Autodesk Inventor part; units mm, degrees
ref_plane "YZ Plane" through (0, 0, 0) normal (1, 0, 0) x (0, 1, 0)
ref_plane "XZ Plane" through (0, 0, 0) normal (0, 1, 0) x (-1, 0, 0)
ref_plane "XY Plane" through (0, 0, 0) normal (0, 0, 1) x (1, 0, 0)
sketch "Sketch1" plane through (0, 0, 0) normal (0, 1, 0) x (-1, 0, 0)
  line L0 (-38.1, 25.4) -> (38.1, 25.4)
  line L1 (38.1, 25.4) -> (38.1, -25.4)
  line L2 (38.1, -25.4) -> (-38.1, -25.4)
  line L3 (-38.1, -25.4) -> (-38.1, 25.4)
  point P0 (0, 0)
  dimension "d0" = 50.8
  dimension "d1" = 76.2
  dimension "d2" = 25.4
  dimension "d3" = 38.1
extrude "Extrusion1" add sketch "Sketch1" along normal blind 25.4
sketch "Sketch2" plane through (38.1, 0, 25.4) normal (1, 0, 0) x (0, 0, -1)
  circle A0 centre (25.4, 38.1) radius 26.9875
  line L0 (0, 0) -> (50.8, 0)
  line L1 (50.8, 0) -> (50.8, 25.4)
  line L2 (0, 25.4) -> (50.8, 25.4)
  line L3 (0, 0) -> (0, 25.4)
  point P0 (25.4, 0)
  dimension "d6" = 53.975
extrude "Extrusion2" cut sketch "Sketch2" against normal through all contours A0 L2 | L2 A0
sketch "Sketch3" plane through (0, 0, 0) normal (0, -1, 0) x (1, 0, 0)
  line L0 (38.1, -25.4) -> (-38.1, -25.4)
  line L1 (19.05, -25.4) -> (-19.05, -25.4)
  line L2 (-19.05, -25.4) -> (-19.05, -38.1)
  line L3 (19.05, -38.1) -> (19.05, -25.4)
  line L4 (12.7, -25.4) -> (-12.7, -25.4)
  line L5 (-12.7, -25.4) -> (-12.7, -31.75)
  line L6 (-12.7, -31.75) -> (12.7, -31.75)
  line L7 (12.7, -31.75) -> (12.7, -25.4)
  line L8 (38.1, -25.4) -> (-38.1, -25.4)
  line L9 (38.1, 25.4) -> (38.1, -25.4)
  line L10 (-38.1, 25.4) -> (38.1, 25.4)
  line L11 (-38.1, -25.4) -> (-38.1, 25.4)
  line L12 (-19.05, -38.1) -> (19.05, -38.1)
  point P0 (0, 0)
  point P1 (12.7, -28.575)
  dimension "d10" = 25.4
  dimension "d11" = 6.35
  dimension "d12" = 6.35
  dimension "d13" = 6.35
  dimension "d14" = 6.35
  dimension "d16" = 12.7
extrude "Extrusion3" add sketch "Sketch3" against normal blind 25.4 contours L3 L12 L2 L0 L5 L6 L7
sketch "Sketch4" plane through (19.05, 0, -25.4) normal (1, 0, 0) x (0, 0, -1)
  line L0 (12.7, 0) -> (0, 0)
  line L1 (12.7, 0) -> (12.7, 25.4)
  line L2 (0, 25.4) -> (12.7, 25.4)
  line L3 (0, 0) -> (0, 25.4)
  arc A0 (-49.2125, 25.4) -> (-1.5875, 25.4) centre (-25.4, 38.1) ccw
  line L4 (-50.8, 25.4) -> (-49.2125, 25.4)
  line L5 (-50.8, 0) -> (-50.8, 25.4)
  line L6 (-50.8, 0) -> (0, 0)
  line L7 (0, 0) -> (0, 25.4)
  line L8 (-1.5875, 25.4) -> (0, 25.4)
  line L9 (6.35, 0) -> (0, 0)
  line L10 (0, 0) -> (12.7, 19.05)
  line L11 (12.7, 0) -> (12.7, 25.4)
  point P0 (-25.4, 0)
  point P1 (12.7, 19.05)
  dimension "d19" = 6.35
extrude "Extrusion4" cut sketch "Sketch4" against normal through all contours L0 L10 L1
mirror "Mirror1" about plane through (0, 0, 0) normal (0, 0, 1) of "Extrusion3", "Extrusion4"
sketch "Sketch5" plane through (0, 0, 0) normal (0, -1, 0) x (1, 0, 0)
  line L0 (-12.7, 25.4) -> (-19.05, 25.4)
  line L1 (-38.1, 25.4) -> (-19.05, 25.4)
  line L2 (-38.1, -25.4) -> (-38.1, 25.4)
  line L3 (-19.05, -25.4) -> (-38.1, -25.4)
  line L4 (-19.05, -25.4) -> (-12.7, -25.4)
  line L5 (12.7, -25.4) -> (-12.7, -25.4)
  line L6 (12.7, -25.4) -> (19.05, -25.4)
  line L7 (38.1, -25.4) -> (19.05, -25.4)
  line L8 (38.1, 25.4) -> (38.1, -25.4)
  line L9 (19.05, 25.4) -> (38.1, 25.4)
  line L10 (19.05, 25.4) -> (12.7, 25.4)
  line L11 (-12.7, 25.4) -> (12.7, 25.4)
  line L12 (38.1, 25.4) -> (38.1, 23.8125)
  line L13 (38.1, 25.4) -> (38.1, 31.75)
  line L14 (19.05, 25.4) -> (38.1, 25.4)
  line L15 (29.0711, 25.4) -> (29.0711, 31.75)
  line L16 (-38.1, -25.4) -> (-38.1, -23.8125)
  line L17 (-38.1, -25.4) -> (-38.1, -31.75)
  line L18 (-23.7998, -25.4) -> (-23.7998, -31.75)
  circle A0 centre (-30.9499, -31.75) radius 3.302
  arc A1 (-38.1, -31.75) -> (-23.7998, -31.75) centre (-30.9499, -31.75) ccw
  point P0 (0, 0)
  dimension "d23" = 14.3002
  dimension "d24" = 6.35
  dimension "d25" = 6.35
  dimension "d26" = 6.604
  dimension "d27" = 6.35
  dimension "d28" = 7.1501
  dimension "d29" = 6.35
extrude "Extrusion5" add sketch "Sketch5" against normal blind 6.35 contours L3 L18 A1 L17
mirror "Mirror2" about plane through (0, 0, 0) normal (0, 0, 1) of "Extrusion5"
equation "\"d12\" = d11"
equation "\"d13\" = d11"
equation "\"d25\" = d24"
equation "\"d27\" = d24"
equation "\"d28\" = 0.5 * d23"
equation "\"d29\" = d24"
properties part number "Part_4_scooter_attachment"
Build history of the part. All positions in model axes, mm. A direction names the side the tool comes from. Round coordinates to 2 decimals unless told otherwise and drop trailing zeros. Write each loop counter-clockwise with the first axis right and the second up, starting at its lowest first coordinate (ties: lowest second). Pieces come first, ordered by that corner, then holes.
1) 3-axis set-ups, long thin cutter, end or side, ignore diameter. For faces 4 (the flat face through (0.267, 11.775, 33.25)), 5 (the flat face through (-12.7, 15, 29)), 6 (the flat face through (-23.8, 3, 29)), 7 (the flat face through (19.05, 15, -30)): which of +Z, -Z, +X, -X, +Y, -Y reach the whole face in a straight line?
2) Drill centre lines: probe 1 along X at (y, z) = (4.25, 31.75); probe 2 along X at (y, z) = (3, -26); probe 3 along X at (y, z) = (9.25, -29). Where is each one in solid material? Low to high.
3) Band-saw the part on D-D, the plane z = 30.5. List the corners of the cut face in (x, y), and give its area (3 significant figures).
4) Band-saw the part on B-B, the plane x = -8. Give the number of separate pieces and of enclosed holes in the cut face, and give its area (3 significant figures).
5) Pin check, flat tips, straight feed: pin 1 (3 mm diameter, centred on y = 16.5, z = -27, fed in from +X); pin 2 (6 mm diameter, centred on x = 8.5, y = 10, fed in from +Z); pin 3 (8 mm diameter, centred on x = 1.5, y = 14, fed in from +Z); pin 4 (5 mm diameter, centred on y = 10.5, z = 27.5, fed in from +X). Stop position of each tip, or through.
6) Mould opens along X. For faces 1 (the flat face through (38.1, 10, 0)), 2 (the flat face through (28, 13, -25.4)), 3 (the flat face through (-12.7, 15, -29)) say: +X half, -X half, draft (parallel to the pull), parting line (faces both ways), or undercut.
7) Band-saw the part on A-A, the plane y = 17.75. List the corners of the cut face in (x, z).
Ans:
1. face 4: +Z, +X, -Y
1. face 5: +Y, -Y
1. face 6: +Z, +Y, -Y
1. face 7: -Z, +X, +Y, -Y
2. probe 1: x = -38.1 to -34.25, -27.65 to -23.8
2. probe 2: x = -38.1 to -23.8, -19.05 to -12.7, 12.7 to 19.05
2. probe 3: x = -19.05 to -12.7, 12.7 to 19.05
3. outline: (-38.1, 0) - (-34.01, 0) - (-34.01, 6.35) - (-38.1, 6.35) - close; (-27.89, 0) - (-23.8, 0) - (-23.8, 6.35) - (-27.89, 6.35) - close; (-19.05, 7.65) - (-12.7, 7.65) - (-12.7, 25.4) - (-19.05, 25.4) - close; (12.7, 7.65) - (19.05, 7.65) - (19.05, 25.4) - (12.7, 25.4) - close
3. area: 277 mm2
4. separate pieces: 3
4. enclosed holes: 0
4. area: 947 mm2
5. pin 1: stops at x = 19.05
5. pin 2: stops at z = 34.07
5. pin 3: stops at z = 37.4
5. pin 4: stops at x = 38.1
6. face 1: +X half
6. face 2: draft
6. face 3: undercut
7. outline: (-38.1, -25.4) - (-19.05, -25.4) - (-19.05, -37.23) - (19.05, -37.23) - (19.05, -25.4) - (38.1, -25.4) - (38.1, -17.73) - (-38.1, -17.73) - close; (-38.1, 17.73) - (38.1, 17.73) - (38.1, 25.4) - (19.05, 25.4) - (19.05, 37.23) - (-19.05, 37.23) - (-19.05, 25.4) - (-38.1, 25.4) - close; hole (-12.7, -31.75) - (12.7, -31.75) - (12.7, -25.4) - (-12.7, -25.4) - close; hole (-12.7, 25.4) - (12.7, 25.4) - (12.7, 31.75) - (-12.7, 31.75) - close
